Verification items for the finished model (mm, model axes). A direction names the side the tool comes from. Give positions to 0.01 mm unless a question says otherwise; leave off trailing zeros. Write each loop counter-clockwise with the first axis right and the second up, starting at its lowest first coordinate (ties: lowest second). Pieces come first, ordered by that corner, then holes.
from build123d import *

# Parameters (mm, degrees)
BOSS_EXTRUDE1_DEPTH   = 15
FILLET1_R             = 5.08
F_5_0MM_DOWEL_HOLE1_D = 5
SKETCH16_R            = 5.5
CUT_EXTRUDE2_DEPTH    = 5
SKETCH14_R            = 2.5
CUT_EXTRUDE1_DEPTH    = 139.704015318
LPATTERN2_COUNT       = 2
LPATTERN2_PITCH       = 49


with BuildPart() as part:
    # Sketch1 → Boss-Extrude1 (new body)
    with BuildSketch(Plane.XY):
        Polygon((27.510468203, 50), (67.924987047, 120), (67.924987047, 81.9), (20.64, 0), (10, -99.432340815), (-10, -99.432340815), (-20.64, 0), (-67.924987047, 81.9), (-67.924987047, 120), (-27.510468203, 50), (-22.510468203, 50), (-22.510468203, 85), (22.510468203, 85), (22.510468203, 50), align=None)
    extrude(amount=BOSS_EXTRUDE1_DEPTH)

    # Fillet1
    # the kernel refuses this fillet: 5.08 mm, written as the material it adds along each edge
    with BuildSketch(Plane(origin=(20.64, 0, 0), x_dir=(0.5000000000000017, 0.8660254037844377, 0), z_dir=(0, 0, 1)), Plane(origin=(-20.64, 0, 0), x_dir=(0.10639999999998911, -0.9943234081524995, 0), z_dir=(0, 0, 1))) as fillet1_piece_1:
        with BuildLine():
            CenterArc((FILLET1_R * 0.211573226201, -FILLET1_R), FILLET1_R, 90, 23.892167456)
            Line((-FILLET1_R * 0.193443374913, -FILLET1_R * 0.0856906689624), (0, 0))
            Line((0, 0), (FILLET1_R * 0.211573226201, 0))
        make_face()
    extrude(amount=15)
    with BuildSketch(Plane(origin=(27.510468203, 50, 0), x_dir=(0.4999999999999992, 0.8660254037844392, 0), z_dir=(0, 0, 1))) as fillet1_piece_2:
        with BuildLine():
            CenterArc((FILLET1_R * 0.57735026919, FILLET1_R), FILLET1_R, 210, 60)
            Line((-FILLET1_R * 0.288675134595, FILLET1_R * 0.5), (0, 0))
            Line((0, 0), (FILLET1_R * 0.57735026919, 0))
        make_face()
    extrude(amount=15)
    with BuildSketch(Plane(origin=(22.510468203, 50, 0), x_dir=(0, 1, 0), z_dir=(0, 0, 1)), Plane(origin=(-22.510468203, 50, 0), x_dir=(-1, 0, 0), z_dir=(0, 0, 1))) as fillet1_piece_3:
        with BuildLine():
            CenterArc((FILLET1_R, -FILLET1_R), FILLET1_R, 90, 90)
            Line((0, -FILLET1_R), (0, 0))
            Line((0, 0), (FILLET1_R, 0))
        make_face()
    extrude(amount=15)
    with BuildSketch(Plane(origin=(-27.510468203, 50, 0), x_dir=(-0.5000000000000053, 0.8660254037844356, 0), z_dir=(0, 0, 1))) as fillet1_piece_4:
        with BuildLine():
            CenterArc((FILLET1_R * 0.57735026919, -FILLET1_R), FILLET1_R, 90, 60)
            Line((-FILLET1_R * 0.288675134595, -FILLET1_R * 0.5), (0, 0))
            Line((0, 0), (FILLET1_R * 0.57735026919, 0))
        make_face()
    extrude(amount=15)
    # the kernel refuses this fillet: 5.08 mm, written as the material it takes off along each edge
    with BuildSketch(Plane(origin=(-10, -99.432340815, -11.413509837), x_dir=(-0.10639999999999113, 0.9943234081524995, 0), z_dir=(0, 0, 1)), Plane(origin=(10, -99.432340815, -11.413509837), x_dir=(-1, 0, 0), z_dir=(0, 0, 1))) as fillet1_2_piece_1:
        with BuildLine():
            CenterArc((FILLET1_R * 0.89870156196, -FILLET1_R), FILLET1_R, 90, 83.892167456)
            Line((-FILLET1_R * 0.0956218461925, -FILLET1_R * 0.8936), (0, 0))
            Line((0, 0), (FILLET1_R * 0.89870156196, 0))
        make_face()
    extrude(amount=37.827019674, mode=Mode.SUBTRACT)
    with BuildSketch(Plane(origin=(67.924987047, 81.9, -3.402954744), x_dir=(-0.4999999999999986, -0.8660254037844396, 0), z_dir=(0, 0, 1)), Plane(origin=(-67.924987047, 81.9, -3.402954744), x_dir=(0, 1, 0), z_dir=(0, 0, 1))) as fillet1_2_piece_2:
        with BuildLine():
            CenterArc((FILLET1_R * 0.267949192431, -FILLET1_R), FILLET1_R, 90, 30)
            Line((-FILLET1_R * 0.232050807569, -FILLET1_R * 0.133974596216), (0, 0))
            Line((0, 0), (FILLET1_R * 0.267949192431, 0))
        make_face()
    extrude(amount=21.805909488, mode=Mode.SUBTRACT)
    with BuildSketch(Plane(origin=(-22.510468203, 85, -12.7), x_dir=(1, 0, 0), z_dir=(0, 0, 1)), Plane(origin=(22.510468203, 85, -12.7), x_dir=(0, -1, 0), z_dir=(0, 0, 1))) as fillet1_2_piece_3:
        with BuildLine():
            CenterArc((FILLET1_R, -FILLET1_R), FILLET1_R, 90, 90)
            Line((0, -FILLET1_R), (0, 0))
            Line((0, 0), (FILLET1_R, 0))
        make_face()
    extrude(amount=40.4, mode=Mode.SUBTRACT)

    # Ø5.0mm Dowel Hole1 (through all)
    with Locations(Plane(origin=(0, 0, 0), x_dir=(-1, 0, 0), z_dir=(0, 0, -1))):
        with Locations((7.5, 15), (-7.5, 15)):
            f_5_0mm_dowel_hole1 = Hole(F_5_0MM_DOWEL_HOLE1_D / 2)

    # Sketch16 → Cut-Extrude2 (cut)
    with BuildSketch(Plane(origin=(0, 0, 0), x_dir=(-1, 0, 0), z_dir=(0, 0, -1))):
        with Locations((-7.5, 15)):
            Circle(SKETCH16_R)
        with Locations((7.5, 15)):
            Circle(SKETCH16_R)
    cut_extrude2 = extrude(amount=-CUT_EXTRUDE2_DEPTH, mode=Mode.SUBTRACT)

    # Sketch14 → Cut-Extrude1 (cut, through all)
    with BuildSketch(Plane.XY.offset(15)):
        with Locations((0, -89.432340815)):
            Circle(SKETCH14_R)
    extrude(amount=-CUT_EXTRUDE1_DEPTH, mode=Mode.SUBTRACT)

    # LPattern2: Ø5.0mm Dowel Hole1, Cut-Extrude2 ×2
    with Locations(*[(0, i * LPATTERN2_PITCH, 0) for i in range(1, LPATTERN2_COUNT)]):
        add(f_5_0mm_dowel_hole1, mode=Mode.SUBTRACT)
        add(cut_extrude2, mode=Mode.SUBTRACT)


solid = part.part
Item 1: Scan lines: line 1 along Y through (x, z) = (7.5, 2.55); line 2 along Y through (x, z) = (7.5, 11.25); line 3 along X through (y, z) = (58.5, 7.5) (3 decimals). Record each from-to range of solid material in increasing order.
Answer key:
line 1: y = -98.99 to 9.5, 20.5 to 58.5, 69.5 to 85
line 2: y = -98.99 to 12.5, 17.5 to 61.5, 66.5 to 85
line 3: x = -54.415 to -32.418, -22.51 to 22.51, 32.418 to 54.415
Item 2: Set-up check for faces 5 (the face through (-6.784, 69.453, 2.465)), 6 (the face through (21.062, 83.472, 7.395)), 7 (the face through (-7.83, 66.48, 10.07)): record each of +Z, -Z, +X, -X, +Y, -Y from which the full face is reachable in a straight line by a thin tool's end or side.
Answer key:
face 5: -Z
face 6: +Z, -Z, +Y
face 7: +Z, -Z
Item 3: Sectioned sample at B-B on y = 98. Record the cut outline in (x, z), then the cut area to 3 significant figures.
Answer key:
outline: (-67.92, 0) - (-55.22, 0) - (-55.22, 15) - (-67.92, 15) - close; (55.22, 0) - (67.92, 0) - (67.92, 15) - (55.22, 15) - close
area: 381 mm2
Item 4: Sectioned sample at C-C on y = 15. Record the cut outline in (x, z).
Answer key:
outline: (-29.3, 0) - (-13, 0) - (-13, 5) - (-10, 5) - (-10, 15) - (-29.3, 15) - close; (-5, 5) - (-2, 5) - (-2, 0) - (2, 0) - (2, 5) - (5, 5) - (5, 15) - (-5, 15) - close; (10, 5) - (13, 5) - (13, 0) - (29.3, 0) - (29.3, 15) - (10, 15) - close
Item 5: Depth check by flat-ended pin: pin 1 (6 mm diameter, centred on y = 75.5, z = 6.5, fed in from -X); pin 2 (5.5 mm diameter, centred on x = -7.5, y = 13, fed in from -Z); pin 3 (3 mm diameter, centred on x = 0, y = -89.43, fed in from +Z); pin 4 (4.5 mm diameter, centred on x = -6, z = 10.5, fed in from +Y). Enter the tip coordinate at first touch or a pass-through.
Answer key:
pin 1: stops at x = -65.96
pin 2: stops at z = 5
pin 3: passes through
pin 4: stops at y = 85
Item 6: Sectioned sample at A-A on z = 7.5. State how many separate pieces and enclosed holes the cut face has, then the cut area to 3 significant figures.
Answer key:
separate pieces: 1
enclosed holes: 5
area: 10,300 mm2
Item 7: Sectioned sample at D-D on y = 64. Record the cut outline in (x, z).
Answer key:
outline: (-57.59, 0) - (-35.59, 0) - (-35.59, 15) - (-57.59, 15) - close; (-22.51, 0) - (-13, 0) - (-13, 5) - (-10, 5) - (-10, 15) - (-22.51, 15) - close; (-5, 5) - (-2, 5) - (-2, 0) - (2, 0) - (2, 5) - (5, 5) - (5, 15) - (-5, 15) - close; (10, 5) - (13, 5) - (13, 0) - (22.51, 0) - (22.51, 15) - (10, 15) - close; (35.59, 0) - (57.59, 0) - (57.59, 15) - (35.59, 15) - close
Item 8: Release check for a two-part mould opening along Y. For faces 1 (the face through (-10, 63, 5)), 2 (the face through (15.576, -47.324, 7.395)), 3 (the face through (-3, 27, 15)), 4 (the face through (5, 14, 5)) record: released by +Y, released by -Y, zero draft, split by the parting line, or undercut.
Answer key:
face 1: undercut
face 2: released by -Y
face 3: zero draft
face 4: undercut
